For this review, use the dimensioned drawing (mm, ordinates from the lowest corner) and the shaded views. Round coordinates to 2 decimals unless told otherwise and drop trailing zeros. Write each loop counter-clockwise with the first axis right and the second up, starting at its lowest first coordinate (ties: lowest second). Pieces come first, ordered by that corner, then holes. Notation, with made-up numbers: M 24.25,68 L 47.25,68 A21 ccw 47.25,75 Z; hole C 23,-1 d1. An arc over 180 degrees is marked long. Answer in a Markdown table with one row per item.
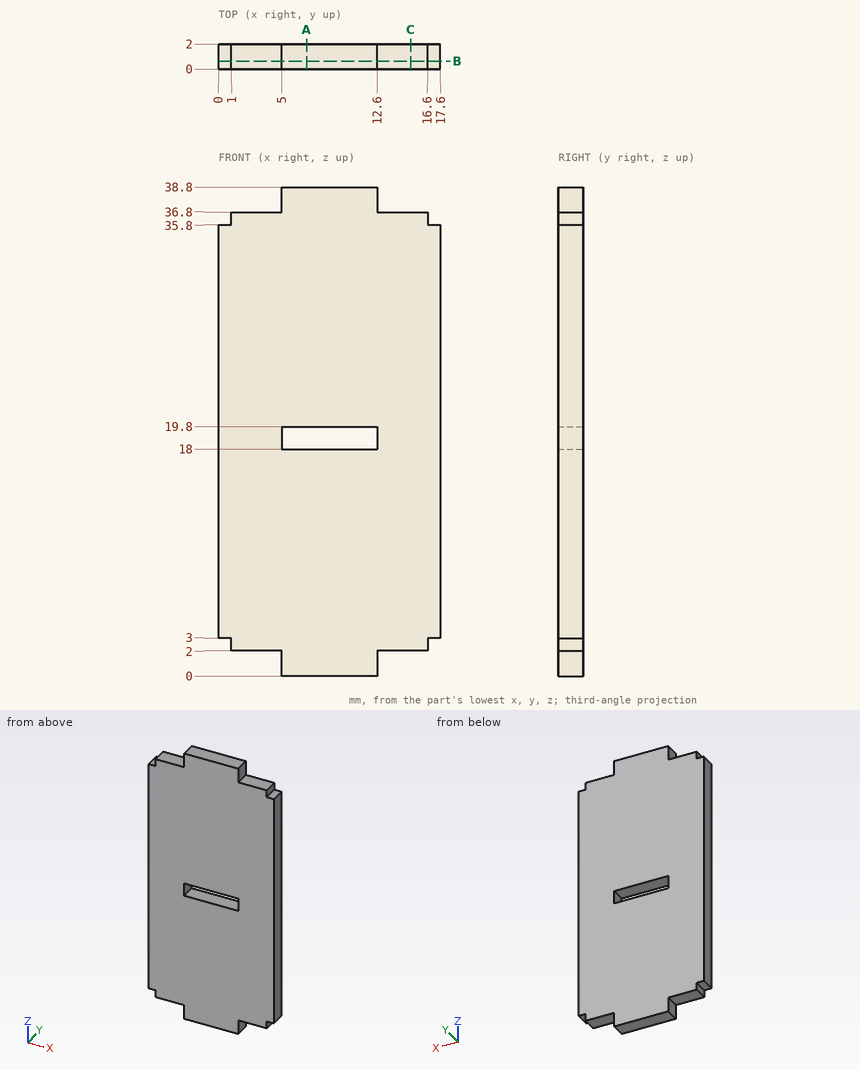
Q1. For probe 1 along Z at (x, y) = (9.5, 1.65); probe 2 along Z at (x, y) = (16, 1.4); probe 3 along X at (y, z) = (1.7, 19.5), list the stretches that pass through material, from the lowest coordinate up.
Found:
| item | result |
|---|---|
| probe 1 | 0 to 18, 19.8 to 38.8 |
| probe 2 | 2 to 36.8 |
| probe 3 | 0 to 5, 12.6 to 17.6 |
Q2. Take a section at C-C (x = 15.25). State the section outline as (y, z) points, then the cut area to 3 significant figures.
Found:
| item | result |
|---|---|
| outline | M 0,2 L 2,2 L 2,36.8 L 0,36.8 Z |
| area | 69.6 mm² |
Q3. Take a section at A-A (x = 7). State the section outline as (y, z) points, then the cut area to 3 significant figures.
Found:
| item | result |
|---|---|
| outline | M 0,0 L 2,0 L 2,18 L 0,18 Z; M 0,19.8 L 2,19.8 L 2,38.8 L 0,38.8 Z |
| area | 74.0 mm² |
Q4. Insertion check: P1, Ø0.5, axis at x = 17.5, y = 1.5, coming from the +Z side; P2, Ø0.6, axis at y = 1, z = 1, coming from the +X side; P3, Ø1.1, axis at x = 0.5, y = 1, coming from the +Z side; P4, Ø0.5, axis at y = 0.5, z = 19, coming from the -X side. Each pin has a flat end and moves straight along its axis. Give the tip position at first contact, or say it passes through.
Found:
| item | result |
|---|---|
| P1 | z = 35.8 |
| P2 | x = 12.6 |
| P3 | z = 36.8 |
| P4 | x = 0 |
Q5. Take a section at B-B (y = 0.65). State the section outline as (x, z) points, then the cut area to 3 significant figures.
Found:
| item | result |
|---|---|
| outline | M 0,3 L 1,3 L 1,2 L 5,2 L 5,0 L 12.6,0 L 12.6,2 L 16.6,2 L 16.6,3 L 17.6,3 L 17.6,35.8 L 16.6,35.8 L 16.6,36.8 L 12.6,36.8 L 12.6,38.8 L 5,38.8 L 5,36.8 L 1,36.8 L 1,35.8 L 0,35.8 Z; hole M 5,18 L 12.6,18 L 12.6,19.8 L 5,19.8 Z |
| area | 625 mm² |
